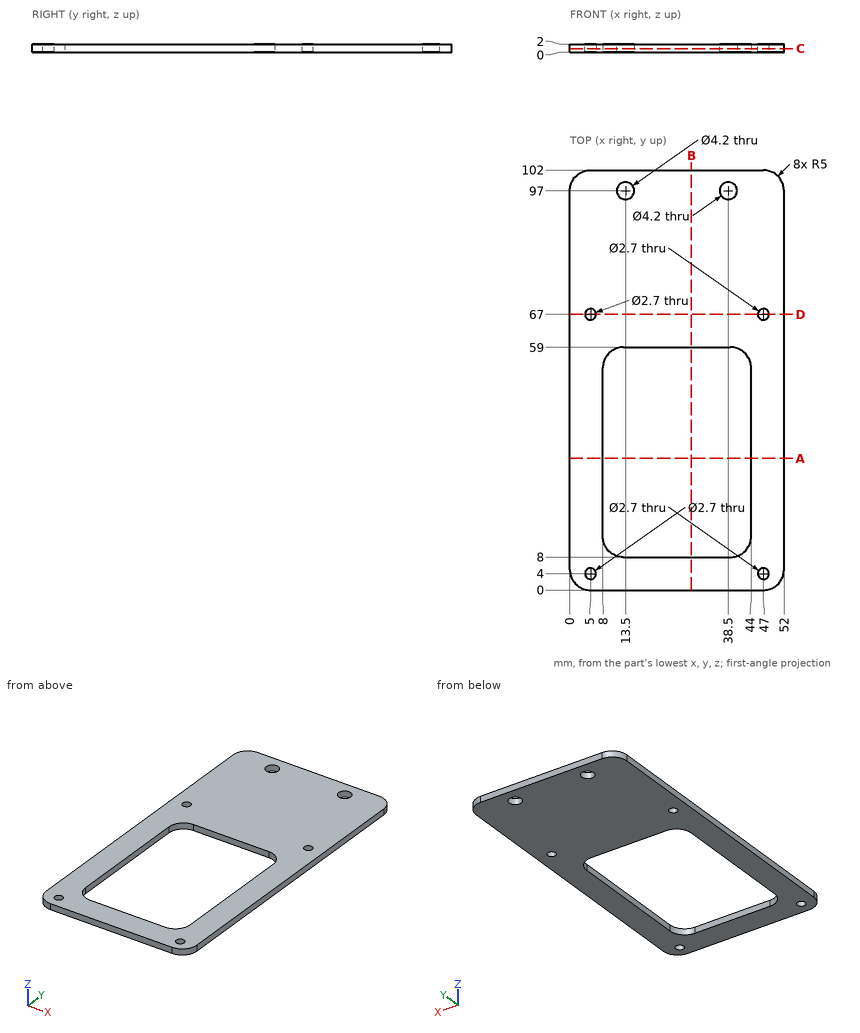
Can you work these out from the drawing? Everything is in mm from the part's minimum corner. Round coordinates to 2 decimals unless told otherwise and drop trailing zeros. Write each loop counter-clockwise with the first axis right and the second up, starting at its lowest first coordinate (ties: lowest second). Pieces come first, ordered by that corner, then holes.
1. Suppose I cut it at D-D (y = 67). List the corners of the cut face in (x, z) for me.
2. Suppose I cut it at C-C (z = 0.9). List the corners of the cut face in (x, y) for me, and give its area (3 significant figures).
3. Suppose I cut it at B-B (x = 29.5). List the corners of the cut face in (y, z) for me.
4. Will this pin go through, and if not, where does the flat tip stop? pin 1 Ø2 at (x, y) = (47, 4) entering from +Z.
5. Suppose I cut it at A-A (y = 32). List the corners of the cut face in (x, z) for me.
6. I need wall thicknesses on L1, parallel to Y at x = 5, z = 1.2; L2, parallel to X at y = 97, z = 0.45; L3, parallel to Y at x = 13.5, z = 1.2. Which ranges of each line are inside material? Lowest first, please.
Answer sheet:
1. outline: (0, 0) - (3.65, 0) - (3.65, 2) - (0, 2) - close; (6.35, 0) - (45.65, 0) - (45.65, 2) - (6.35, 2) - close; (48.35, 0) - (52, 0) - (52, 2) - (48.35, 2) - close
2. outline: (0, 5) arc R5 ccw to (5, 0) - (47, 0) arc R5 ccw to (52, 5) - (52, 97) arc R5 ccw to (47, 102) - (5, 102) arc R5 ccw to (0, 97) - close; hole circle Ø2.7 at (5, 4); hole circle Ø2.7 at (5, 67); hole (8, 13) arc R5 ccw to (13, 8) - (39, 8) arc R5 ccw to (44, 13) - (44, 54) arc R5 ccw to (39, 59) - (13, 59) arc R5 ccw to (8, 54) - close; hole circle Ø4.2 at (13.5, 97); hole circle Ø4.2 at (38.5, 97); hole circle Ø2.7 at (47, 4); hole circle Ø2.7 at (47, 67)
2. area: 3,420 mm2
3. outline: (0, 0) - (8, 0) - (8, 2) - (0, 2) - close; (59, 0) - (102, 0) - (102, 2) - (59, 2) - close
4. pin 1: passes through
5. outline: (0, 0) - (8, 0) - (8, 2) - (0, 2) - close; (44, 0) - (52, 0) - (52, 2) - (44, 2) - close
6. L1: y = 0 to 2.65, 5.35 to 65.65, 68.35 to 102
6. L2: x = 0 to 11.4, 15.6 to 36.4, 40.6 to 52
6. L3: y = 0 to 8, 59 to 94.9, 99.1 to 102
